from build123d import *

# Parameters (mm, degrees)
Y_KSEKLIK_EKSTR_ZYON1_DEPTH      = 3
Y_KSEKLIK_EKSTR_ZYON1_DEPTH_BACK = 3
Y_KSEKLIK_EKSTR_ZYON7_DEPTH      = 1.5
Y_KSEKLIK_EKSTR_ZYON7_DEPTH_BACK = 1.5
IZIM11_R                         = 1
Y_KSEKLIK_EKSTR_ZYON8_DEPTH      = 2
Y_KSEKLIK_EKSTR_ZYON8_DEPTH_BACK = 3
RADYUS3_R                        = 0.3
IZIM12_R                         = 1.75
Y_KSEKLIK_EKSTR_ZYON9_DEPTH      = 1
RADYUS4_R                        = 0.3
KES_EKSTR_ZYON5_DEPTH            = 0.2
IZIM14_R                         = 0.25
Y_KSEKLIK_EKSTR_ZYON10_DEPTH     = 3


with BuildPart() as part:
    # izim1 → Y_kseklik-Ekstr_zyon1 (new body, two sides)
    with BuildSketch(Plane.XY) as y_kseklik_ekstr_zyon1_sk:
        with BuildLine():
            Line((-1.5, 2.5), (1.5, 2.5))
            ThreePointArc((1.5, 2.5), (1.853553391, 2.353553391), (2, 2))
            Line((2, 2), (2, -2))
            ThreePointArc((2, -2), (1.853553391, -2.353553391), (1.5, -2.5))
            Line((1.5, -2.5), (-1.5, -2.5))
            ThreePointArc((-1.5, -2.5), (-1.853553391, -2.353553391), (-2, -2))
            Line((-2, -2), (-2, 2))
            ThreePointArc((-2, 2), (-1.853553391, 2.353553391), (-1.5, 2.5))
        make_face()
        with BuildLine():
            Line((-1.8, 2), (-1.8, -2))
            ThreePointArc((-1.8, -2), (-1.712132034, -2.212132034), (-1.5, -2.3))
            Line((-1.5, -2.3), (1.5, -2.3))
            ThreePointArc((1.5, -2.3), (1.712132034, -2.212132034), (1.8, -2))
            Line((1.8, -2), (1.8, 2))
            ThreePointArc((1.8, 2), (1.712132034, 2.212132034), (1.5, 2.3))
            Line((1.5, 2.3), (-1.5, 2.3))
            ThreePointArc((-1.5, 2.3), (-1.712132034, 2.212132034), (-1.8, 2))
        make_face(mode=Mode.SUBTRACT)
    extrude(amount=Y_KSEKLIK_EKSTR_ZYON1_DEPTH)
    extrude(y_kseklik_ekstr_zyon1_sk.sketch, amount=-Y_KSEKLIK_EKSTR_ZYON1_DEPTH_BACK)



with BuildPart() as body_2:
    # izim10 → Y_kseklik-Ekstr_zyon7 (new body, two sides)
    with BuildSketch(Plane(origin=(0, 0, 0), x_dir=(0, 0, -1), z_dir=(1, 0, 0))) as y_kseklik_ekstr_zyon7_sk:
        with BuildLine():
            Line((-2.684933096, 0), (-2.648317711, -0.196619718))
            add(Edge.make_bspline(
                [(-2.648317711, -0.196619718), (-0.912612771, 0.126610857), (0.912612771, 0.126610857), (2.648317711, -0.196619718)],
                knots=[0, 0, 0, 0, 1, 1, 1, 1], degree=3))
            Line((2.648317711, -0.196619718), (2.684933096, 0))
            add(Edge.make_bspline(
                [(-2.684933096, 0), (-0.894977699, 0.333333333), (0.894977699, 0.333333333), (2.684933096, 0)],
                knots=[0, 0, 0, 0, 1, 1, 1, 1], degree=3))
        make_face()
    extrude(amount=Y_KSEKLIK_EKSTR_ZYON7_DEPTH)
    extrude(y_kseklik_ekstr_zyon7_sk.sketch, amount=-Y_KSEKLIK_EKSTR_ZYON7_DEPTH_BACK)


with BuildPart() as part_1:
    add(part.part)

    add(body_2.part)  # Y_kseklik-Ekstr_zyon8 merges body 2
    # izim11 → Y_kseklik-Ekstr_zyon8 (add, two sides)
    with BuildSketch(Plane(origin=(0, 2.5, 0), x_dir=(1, 0, 0), z_dir=(0, 1, 0))) as y_kseklik_ekstr_zyon8_sk:
        Circle(IZIM11_R)
    extrude(amount=Y_KSEKLIK_EKSTR_ZYON8_DEPTH)
    extrude(y_kseklik_ekstr_zyon8_sk.sketch, amount=-Y_KSEKLIK_EKSTR_ZYON8_DEPTH_BACK)

    # Radyus3
    radyus3_edges = [part_1.edges().sort_by_distance(p)[0] for p in [
        (-1, -0.5, 0),
    ]]
    fillet(radyus3_edges, radius=RADYUS3_R)

    # izim12 → Y_kseklik-Ekstr_zyon9 (add)
    with BuildSketch(Plane(origin=(0, 4.5, 0), x_dir=(1, 0, 0), z_dir=(0, 1, 0))):
        Circle(IZIM12_R)
    extrude(amount=Y_KSEKLIK_EKSTR_ZYON9_DEPTH)

    # Radyus4
    radyus4_edges = [part_1.edges().sort_by_distance(p)[0] for p in [
        (-1.75, 5.5, 0),
    ]]
    fillet(radyus4_edges, radius=RADYUS4_R)

    # izim13 → Kes-Ekstr_zyon5 (cut)
    with BuildSketch(Plane(origin=(0, 5.5, 0), x_dir=(1, 0, 0), z_dir=(0, 1, 0))):
        Polygon((-0.25, -0.25), (-0.25, -2.096616873), (0.25, -2.096616873), (0.25, -0.25), (2.70967232, -0.25), (2.70967232, 0.25), (0.25, 0.25), (0.25, 2.096616873), (-0.25, 2.096616873), (-0.25, 0.25), (-2.70967232, 0.25), (-2.70967232, -0.25), align=None)
    extrude(amount=-KES_EKSTR_ZYON5_DEPTH, mode=Mode.SUBTRACT)

    # izim14 → Y_kseklik-Ekstr_zyon10 (add)
    with BuildSketch(Plane.XZ.offset(2.5)):
        Circle(IZIM14_R)
    extrude(amount=Y_KSEKLIK_EKSTR_ZYON10_DEPTH)

    # izim15 → D_nd_r2 (revolve)
    with BuildSketch(Plane(origin=(0, 0, 0), x_dir=(0, 0, -1), z_dir=(1, 0, 0))):
        with BuildLine():
            Line((0, -5.5), (0, -4.5))
            Line((0, -4.5), (1, -4.5))
            add(Edge.make_bspline(
                [(0, -5.5), (0.812408403, -5.158653256), (1, -4.5)],
                knots=[0, 0, 0, 0.79847646, 0.79847646, 0.79847646], degree=2))
        make_face()
    revolve(axis=Axis((0, -5.5, 0), (0, 1, 0)))


solid = part_1.part
Source: CAD feature listing. Evaluate the final solid. Frame: model axes, mm. A direction names the side the tool comes from. Give positions to 0.01 mm unless a question says otherwise; leave off trailing zeros. Order: outer loops, then holes, each group sorted by start corner. A loop starts at its lowest first (then second) coordinate and runs counter-clockwise, first axis right, second up. Notation, with made-up numbers: (-2, -38) -> (15, -38) arc R20 ccw to (15, -33) -> close; hole circle Ø11 at (81.25, 16.25). An arc over 180 degrees is marked (long way). Use a Markdown table: item, result.
1) Section query C-C, the plane y = -3. Return the cut outline in (x, z).
Answer list:
| item | result |
|---|---|
| outline | circle Ø0.5 at (0, 0) |
2) Section query A-A, the plane y = 1.75. Return the cut outline in (x, z).
Answer list:
| item | result |
|---|---|
| outline | (-2, -3) -> (-1.8, -3) -> (-1.8, 3) -> (-2, 3) -> close; circle Ø2 at (0, 0); (1.8, -3) -> (2, -3) -> (2, 3) -> (1.8, 3) -> close |
3) Contact query for a flat-ended pin moving along its axis: P1, Ø2, axis at x = 1, y = -4, coming from the +Z side. Output: stop coordinate, or through.
Answer list:
| item | result |
|---|---|
| P1 | z = 0.99 |
4) Mould query, pull axis Z, two halves, no side actions, for faces 4 (the flat face through (0, -2.3, 0)), 5 (the cylindrical face through (0, 1, 1)), 6 (the flat face through (0, 5.3, 0)). Classes: +Z half, -Z half, draft (parallel to the pull), parting line (faces both ways), or undercut.
Answer list:
| item | result |
|---|---|
| face 4 | draft |
| face 5 | parting line |
| face 6 | undercut |
5) Ray query, line 1 along Y through (x, z) = (-0.3, -1.4); line 2 along Y through (x, z) = (0.2, -1.35); line 3 along Y through (x, z) = (0.3, -1.8). Return the intervals inside material, ascending. Write a range as [from, to].
Answer list:
| item | result |
|---|---|
| line 1 | [-2.5, -2.3], [-0.02, 0.18], [2.3, 2.5], [4.5, 5.5] |
| line 2 | [-2.5, -2.3], [-0.02, 0.19], [2.3, 2.5], [4.5, 5.3] |
| line 3 | [-2.5, -2.3], [-0.07, 0.14], [2.3, 2.5] |
6) Reachability of faces 1 (the cylindrical face through (1.617, 4.845, 0.67)), 2 (the flat face through (0, -0.5, 0)), 3 (the flat face through (1, 2.3, 1)) from +Z, -Z, +X, -X, +Y, -Y: full face, straight path, thin tool, end or side. Return the list, or none.
Answer list:
| item | result |
|---|---|
| face 1 | +Y |
| face 2 | +Z, -Z |
| face 3 | none |
7) Section query B-B, the plane x = 0.4. Count the separate pieces of the cut face and the enclosed holes in it, then the cut area to 3 significant figures.
Answer list:
| item | result |
|---|---|
| separate pieces | 3 |
| enclosed holes | 0 |
| area | 16.2 mm² |
